Build history of the part. All positions in model axes, mm. A direction names the side the tool comes from. Round coordinates to 2 decimals unless told otherwise and drop trailing zeros. Loops run counter-clockwise (first coordinate to the right, second up) from the corner with the lowest first, then second, coordinate; pieces in that order, holes last. Notation, with made-up numbers: M 10,65.5 L 16,65.5 A30 ccw 16,99.5 Z; hole C 39,27.25 d11. An arc over 180 degrees is marked long. Use one line per item in the form item = value. Start each with the question number.
```python
from build123d import *

# Parameters (mm, degrees)
SKETCH1_R           = 6
BOSS_EXTRUDE2_DEPTH = 12
SKETCH2_W           = 12
SKETCH2_H           = 100
BOSS_EXTRUDE3_DEPTH = 60
SKETCH3_R           = 6
CUT_EXTRUDE1_DEPTH  = 341.65676581


with BuildPart() as part:
    # Sketch1 → Boss-Extrude2 (new body)
    with BuildSketch(Plane(origin=(0, 0, 0), x_dir=(1, 0, 0), z_dir=(0, 1, 0))):
        with BuildLine():
            Line((550, 175), (550, 75))
            Line((550, 75), (443.705983732, 75))
            ThreePointArc((443.705983732, 75), (450, 0), (443.705983732, -75))
            Line((443.705983732, -75), (550, -75))
            Line((550, -75), (550, -175))
            Line((550, -175), (414.578098794, -175))
            ThreePointArc((414.578098794, -175), (393.796888861, -217.770545124), (368.61841993, -258.109396358))
            Line((368.61841993, -258.109396358), (327.660817716, -229.43057454))
            ThreePointArc((327.660817716, -229.43057454), (400, 0), (327.660817716, 229.43057454))
            Line((327.660817716, 229.43057454), (368.61841993, 258.109396358))
            ThreePointArc((368.61841993, 258.109396358), (393.796888861, 217.770545124), (414.578098794, 175))
            Line((414.578098794, 175), (550, 175))
        make_face()
        with Locations(Location((368.060796608, -212.5, 0), (0, 0, 270))):
            Circle(SKETCH1_R, mode=Mode.SUBTRACT)
        with Locations(Location((425, 0, 0), (0, 0, 270))):
            Circle(SKETCH1_R, mode=Mode.SUBTRACT)
        with Locations(Location((368.060796608, 212.5, 0), (0, 0, 270))):
            Circle(SKETCH1_R, mode=Mode.SUBTRACT)
    extrude(amount=BOSS_EXTRUDE2_DEPTH)

    # Sketch2 → Boss-Extrude3 (add)
    with BuildSketch(Plane(origin=(0, 12, 0), x_dir=(1, 0, 0), z_dir=(0, 1, 0))):
        with Locations((544, 125)):
            Rectangle(SKETCH2_W, SKETCH2_H)
        with Locations((544, -125)):
            Rectangle(SKETCH2_W, SKETCH2_H)
    extrude(amount=BOSS_EXTRUDE3_DEPTH)

    # Sketch3 → Cut-Extrude1 (cut, through all)
    with BuildSketch(Plane.ZY.offset(-538)):
        with Locations((-150, 42)):
            Circle(SKETCH3_R)
        with Locations((-100, 42)):
            Circle(SKETCH3_R)
        with Locations((100, 42)):
            Circle(SKETCH3_R)
        with Locations((150, 42)):
            Circle(SKETCH3_R)
    extrude(amount=-CUT_EXTRUDE1_DEPTH, mode=Mode.SUBTRACT)


solid = part.part
```
Q1. Saw through at A-A (z = 0). Give the cut face in (x, y), and give its area (3 significant figures).
Q2. Saw through at B-B (y = 20). Give the cut face in (x, z), and give its area (3 significant figures).
Q3. Pull direction Z, two halves, no side cores. Call faces 4 (the face through (550, 35, -124)), 5 (the face through (348.426, 5.916, 243.971)), 6 (the face through (543.92, 38.35, 145.24)), 7 (the face through (497, 11.8, -175)): pulls with the +Z half, pulls with the -Z half, needs draft (parallel to the pull), parting line crosses it, or undercut.
Q4. Drop flat-ended pins along their axis: P1, Ø15.5, axis at x = 368.06, z = 212.5, coming from the +Y side; P2, Ø18, axis at y = 50, z = -138, coming from the -X side; P3, Ø15.5, axis at y = 42, z = -100, coming from the +X side; P4, Ø9.5, axis at x = 425, z = 0, coming from the +Y side. Give the stop position or say it passes through.
Q5. Saw through at C-C (y = 42). Give the cut face in (x, z), and give its area (3 significant figures).
Q6. Saw through at D-D (z = 100). Give the cut face in (x, y), and give its area (3 significant figures).
Q7. Wall check: probe 1 along Y at (x, z) = (544, -150); probe 2 along Z at (x, y) = (516, 8); probe 3 along Z at (x, y) = (425, 7.25). Give the ranges that are in metal, low to high.
Q8. Tool access for faces 1 (the face through (434, 12, 54)), 2 (the face through (512.4, 11.8, -75)), 3 (the face through (544, 42, 94)): list every direction of +Z, -Z, +X, -X, +Y, -Y with a clear straight run to the whole face (end or side of a thin tool).
Filled in:
q1.outline = M 400,0 L 419,0 L 419,12 L 400,12 Z; M 431,0 L 450,0 L 450,12 L 431,12 Z
q1.area = 456 mm²
q2.outline = M 538,-175 L 550,-175 L 550,-75 L 538,-75 Z; M 538,75 L 550,75 L 550,175 L 538,175 Z
q2.area = 2,400 mm²
q3.face_4 = needs draft
q3.face_5 = pulls with the +Z half
q3.face_6 = undercut
q3.face_7 = pulls with the -Z half
q4.P1 = 12
q4.P2 = 538
q4.P3 = 550
q4.P4 = through
q5.outline = M 538,-175 L 550,-175 L 550,-156 L 538,-156 Z; M 538,-144 L 550,-144 L 550,-106 L 538,-106 Z; M 538,-94 L 550,-94 L 550,-75 L 538,-75 Z; M 538,75 L 550,75 L 550,94 L 538,94 Z; M 538,106 L 550,106 L 550,144 L 538,144 Z; M 538,156 L 550,156 L 550,175 L 538,175 Z
q5.area = 1,820 mm²
q6.outline = M 387.3,0 L 550,0 L 550,36 L 538,36 L 538,12 L 387.3,12 Z; M 538,48 L 550,48 L 550,72 L 538,72 Z
q6.area = 2,530 mm²
q7.probe_1 = 0 to 36, 48 to 72
q7.probe_2 = -175 to -75, 75 to 175
q7.probe_3 = -175 to -6, 6 to 175
q8.face_1 = +Z, -Z, -X, +Y
q8.face_2 = +X, +Y, -Y
q8.face_3 = +X, -X
